Build history of the part. All positions in model axes, mm. A direction names the side the tool comes from. Round coordinates to 2 decimals unless told otherwise and drop trailing zeros. Write each loop counter-clockwise with the first axis right and the second up, starting at its lowest first coordinate (ties: lowest second). Pieces come first, ordered by that corner, then holes. Notation, with made-up numbers: (-32.5, 66.25) - (-28.5, 66.25) arc R19 ccw to (-28.5, 97.25) - close; hole circle Ø9 at (-31, 23). An arc over 180 degrees is marked (long way). Answer as a JSON object with one key per item and string values. Group by question number.
Item 1: Slice it at B-B, the plane z = 3.5. List the corners of the cut face in (x, y), then the cut area to 3 significant figures.
Item 2: Slice it at A-A, the plane y = 2. List the corners of the cut face in (x, z), then the cut area to 3 significant figures.
Item 3: Flat gauge pins, fed straight in: pin 1 (2.5 mm diameter, centred on x = 6, z = 0, fed in from -Y); pin 2 (1 mm diameter, centred on x = 5.5, y = -14, fed in from +Z); pin 3 (1.6 mm diameter, centred on x = 6, y = 0, fed in from +Z). Where does each tip first touch, or does it go through?
Item 4: Slice it at D-D, the plane x = 13.25. List the corners of the cut face in (y, z).
Item 5: Probe line 1 (X direction, y = 16, z = 9); line 2 (Z direction, x = 6, y = -16.4) (3 decimals); line 3 (X direction, y = -16.9, z = 0) (3 decimals). List the from-to ranges inside material, lowest first. Write a range as from..to.
Item 6: Two-plate mould, pull along Y, no slides. Class faces 6 (the cylindrical face through (12.928, 18.548, -4.119)), 7 (the cylindrical face through (7, -0.22, -15.43)), 8 (the conical face through (6.158, -0.082, -12.504)), 9 (the cylindrical face through (5, -15.89, -0.22)): +Y half, -Y half, draft (parallel to the pull), parting line (faces both ways), or undercut.
Item 7: Slice it at C-C, the plane x = 3.5. List the corners of the cut face in (y, z), then the cut area to 3 significant figures.
Item 8: Which spindle directions (+Z, -Z, +X, -X, +Y, -Y) get a long thin tool onto all of the face, cutting with end or side? Do faces 1 (the flat face through (15.97, 0, 0)), 2 (the flat face through (0, 0, 0)), 3 (the cylindrical face through (4.915, -5.38, 17.085)), 4 (the cylindrical face through (5, 15.43, 0.22)), 5 (the cylindrical face through (7.024, 0.045, 15.885)). Say none if no direction does.
from build123d import *

# Parameters (mm, degrees)
M2_5_TAPPED_HOLE1_D               = 2.05
M2_5_TAPPED_HOLE1_DEPTH           = 4
M2_5_TAPPED_HOLE1_TIP             = 0.615882135
M2_5_TAPPED_HOLE1_ON_FACE_2_D     = 2.05
M2_5_TAPPED_HOLE1_ON_FACE_2_DEPTH = 4
M2_5_TAPPED_HOLE1_ON_FACE_2_TIP   = 0.615882135
M2_5_TAPPED_HOLE1_ON_FACE_3_D     = 2.05
M2_5_TAPPED_HOLE1_ON_FACE_3_DEPTH = 4
M2_5_TAPPED_HOLE1_ON_FACE_3_TIP   = 0.615882135
M2_5_TAPPED_HOLE2_D               = 2.05
M2_5_TAPPED_HOLE2_DEPTH           = 4.9
M2_5_TAPPED_HOLE2_TIP             = 0.615882135
M2_5_TAPPED_HOLE2_ON_FACE_2_D     = 2.05
M2_5_TAPPED_HOLE2_ON_FACE_2_DEPTH = 4.9
M2_5_TAPPED_HOLE2_ON_FACE_2_TIP   = 0.615882135


with BuildPart() as part:
    # Sketch1 → Revolve1 (revolve)
    with BuildSketch(Plane.XY, mode=Mode.PRIVATE) as revolve1_sk:
        Polygon((0, 17.8825346), (0, 0), (15.97, 0), (15.97, 17), (15.97, 19), (9.97, 19), (9.97, 17.9125346), (0, 17.9125346), align=None)
    revolve(revolve1_sk.sketch.rotate(Axis((-76.24269061, 0, 0), (1, 0, 0)), 90), axis=Axis((-76.24269061, 0, 0), (1, 0, 0)))

    # M2.5 Tapped Hole1
    with Locations(Plane(origin=(6, -17.9125346, 0), x_dir=(0, 0, -1), z_dir=(0, -1, 0))):
        with Locations((0, 0)):
            Hole(M2_5_TAPPED_HOLE1_D / 2, depth=M2_5_TAPPED_HOLE1_DEPTH)
            with Locations((0, 0, -(M2_5_TAPPED_HOLE1_DEPTH + M2_5_TAPPED_HOLE1_TIP / 2))):  # 118° drill point
                Cone(0, M2_5_TAPPED_HOLE1_D / 2, M2_5_TAPPED_HOLE1_TIP, mode=Mode.SUBTRACT)

    # M2.5 Tapped Hole1 on face 2
    with Locations(Plane(origin=(6, 0, 17.9125346), x_dir=(1, 0, 0), z_dir=(0, 0, 1))):
        with Locations((0, 0)):
            Hole(M2_5_TAPPED_HOLE1_ON_FACE_2_D / 2, depth=M2_5_TAPPED_HOLE1_ON_FACE_2_DEPTH)
            with Locations((0, 0, -(M2_5_TAPPED_HOLE1_ON_FACE_2_DEPTH + M2_5_TAPPED_HOLE1_ON_FACE_2_TIP / 2))):  # 118° drill point
                Cone(0, M2_5_TAPPED_HOLE1_ON_FACE_2_D / 2, M2_5_TAPPED_HOLE1_ON_FACE_2_TIP, mode=Mode.SUBTRACT)

    # M2.5 Tapped Hole1 on face 3
    with Locations(Plane(origin=(-38.298616193, 0, -8.034883706), x_dir=(0, 0, -1), z_dir=(0, -1, 0))):
        with Locations((0, 0)):
            Hole(M2_5_TAPPED_HOLE1_ON_FACE_3_D / 2, depth=M2_5_TAPPED_HOLE1_ON_FACE_3_DEPTH)
            with Locations((0, 0, -(M2_5_TAPPED_HOLE1_ON_FACE_3_DEPTH + M2_5_TAPPED_HOLE1_ON_FACE_3_TIP / 2))):  # 118° drill point
                Cone(0, M2_5_TAPPED_HOLE1_ON_FACE_3_D / 2, M2_5_TAPPED_HOLE1_ON_FACE_3_TIP, mode=Mode.SUBTRACT)

    # M2.5 Tapped Hole2
    with Locations(Plane(origin=(6, 0, -17.9125346), x_dir=(0, -1, 0), z_dir=(0, 0, -1))):
        with Locations((0, 0)):
            Hole(M2_5_TAPPED_HOLE2_D / 2, depth=M2_5_TAPPED_HOLE2_DEPTH)
            with Locations((0, 0, -(M2_5_TAPPED_HOLE2_DEPTH + M2_5_TAPPED_HOLE2_TIP / 2))):  # 118° drill point
                Cone(0, M2_5_TAPPED_HOLE2_D / 2, M2_5_TAPPED_HOLE2_TIP, mode=Mode.SUBTRACT)

    # M2.5 Tapped Hole2 on face 2
    with Locations(Plane(origin=(6, 17.9125346, 0), x_dir=(0, 0, 1), z_dir=(0, 1, 0))):
        with Locations((0, 0)):
            Hole(M2_5_TAPPED_HOLE2_ON_FACE_2_D / 2, depth=M2_5_TAPPED_HOLE2_ON_FACE_2_DEPTH)
            with Locations((0, 0, -(M2_5_TAPPED_HOLE2_ON_FACE_2_DEPTH + M2_5_TAPPED_HOLE2_ON_FACE_2_TIP / 2))):  # 118° drill point
                Cone(0, M2_5_TAPPED_HOLE2_ON_FACE_2_D / 2, M2_5_TAPPED_HOLE2_ON_FACE_2_TIP, mode=Mode.SUBTRACT)


solid = part.part
Geometry says:
{
 "1": {"outline": "(0, -17.57) - (9.97, -17.57) - (9.97, -18.67) - (15.97, -18.67) - (15.97, 18.67) - (9.97, 18.67) - (9.97, 17.57) - (0, 17.57) - close", "area": "574 mm^2"},
 "2": {"outline": "(0, -17.8) - (9.97, -17.8) - (9.97, -18.89) - (15.97, -18.89) - (15.97, 18.89) - (9.97, 18.89) - (9.97, 17.8) - (0, 17.8) - close", "area": "582 mm^2"},
 "3": {"pin 1": "stops at y = -17.91", "pin 2": "stops at z = 11.77", "pin 3": "stops at z = 13.78"},
 "4": {"outline": "circle Ø38 at (0, 0)"},
 "5": {"line 1": "x = 9.97..15.97", "line 2": "z = -7.204..-1.025, 1.025..7.204", "line 3": "x = 0..4.975, 7.025..15.97"},
 "6": {"face 6": "parting line", "face 7": "undercut", "face 8": "undercut", "face 9": "draft"},
 "7": {"outline": "circle Ø35.83 at (0, 0)", "area": "1,010 mm^2"},
 "8": {"face 1": "+Z, -Z, +X, +Y, -Y", "face 2": "+Z, -Z, -X, +Y, -Y", "face 3": "-X", "face 4": "+Y", "face 5": "+Z"}
}
